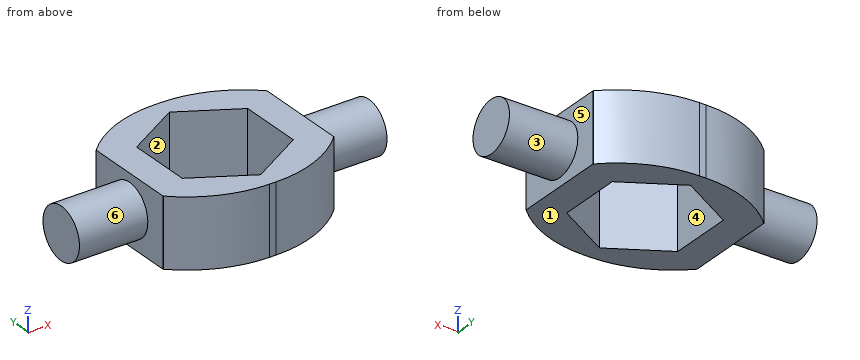
from build123d import *

# Parameters (mm, degrees)
SKETCH1_W           = 63.5
SKETCH1_H           = 60.360264722
BOSS_EXTRUDE1_DEPTH = 25.4
CHAMFER1_SIZE       = 12.7
SKETCH2_R           = 9.525
BOSS_EXTRUDE2_DEPTH = 25.4
FILLET1_R           = 43.18


with BuildPart() as part:
    # Sketch1 → Boss-Extrude1 (new body)
    with BuildSketch(Plane.XY):
        with Locations((31.75, 30.180132361)):
            Rectangle(SKETCH1_W, SKETCH1_H)
        Polygon((11.1125, 42.095198541), (11.1125, 18.26506618), (31.75, 6.35), (52.3875, 18.26506618), (52.3875, 42.095198541), (31.75, 54.010264722), align=None, mode=Mode.SUBTRACT)
    extrude(amount=BOSS_EXTRUDE1_DEPTH)

    # Chamfer1
    chamfer1_edges = [part.edges().sort_by_distance(p)[0] for p in [
        (0, 60.360264722, 12.7),
        (63.5, 60.360264722, 12.7),
        (63.5, 0, 12.7),
        (0, 0, 12.7),
    ]]
    chamfer(chamfer1_edges, length=CHAMFER1_SIZE)

    # Sketch2 → Boss-Extrude2 (add)
    with BuildSketch(Plane.ZY):
        with Locations((12.7, 30.180132361)):
            Circle(SKETCH2_R)
    boss_extrude2 = extrude(amount=BOSS_EXTRUDE2_DEPTH)

    # Mirror1: Boss-Extrude2 across plane
    add(boss_extrude2.mirror(Plane(origin=(31.75, 0, 0), x_dir=(0, 0, 1), z_dir=(1, 0, 0))))

    # Fillet1
    fillet1_edges = [part.edges().sort_by_distance(p)[0] for p in [
        (12.7, 60.360264722, 12.7),
        (50.8, 60.360264722, 12.7),
        (12.7, 0, 12.7),
        (50.8, 0, 12.7),
    ]]
    fillet(fillet1_edges, radius=FILLET1_R)


solid = part.part
Can you work these out from the model? Positions are in its coordinate system, mm. Face numbers are marked on the shaded views. A direction names the side the tool comes from. Give positions to 0.01 mm unless a question says otherwise; leave off trailing zeros. Loops run counter-clockwise (first coordinate to the right, second up) from the corner with the lowest first, then second, coordinate; pieces in that order, holes last. Notation, with made-up numbers: (37, -38) - (96, -38) arc R32 cw to (96, -8) - close; hole circle Ø11 at (-11.5, 52). An arc over 180 degrees is marked (long way). Return JSON: item names as keys, results as strings.
1. I want a section at B-B on x = 37. Please give me the cut outline in (y, z).
Output values:
{"outline": "(0.19, 0) - (9.38, 0) - (9.38, 25.4) - (0.19, 25.4) - close; (50.98, 0) - (60.17, 0) - (60.17, 25.4) - (50.98, 25.4) - close"}
2. I want a section at C-C on y = 25. Please give me the cut outline in (x, z), and give its area (3 significant figures).
Output values:
{"outline": "(-25.4, 4.71) - (0, 4.71) - (0, 0) - (11.11, 0) - (11.11, 25.4) - (0, 25.4) - (0, 20.69) - (-25.4, 20.69) - close; (52.39, 0) - (63.5, 0) - (63.5, 4.71) - (88.9, 4.71) - (88.9, 20.69) - (63.5, 20.69) - (63.5, 25.4) - (52.39, 25.4) - close", "area": "1,380 mm²"}
3. I want a section at D-D on z = 23.5. Please give me the cut outline in (x, y), and give its area (3 significant figures).
Output values:
{"outline": "(0, 12.7) - (0.05, 12.65) arc R43.18 ccw to (30.59, 0) - (32.91, 0) arc R43.18 ccw to (63.45, 12.65) - (63.5, 12.7) - (63.5, 47.66) - (63.45, 47.71) arc R43.18 ccw to (32.91, 60.36) - (30.59, 60.36) arc R43.18 ccw to (0.05, 47.71) - (0, 47.66) - close; hole (11.11, 18.27) - (31.75, 6.35) - (52.39, 18.27) - (52.39, 42.1) - (31.75, 54.01) - (11.11, 42.1) - close", "area": "1,870 mm²"}
4. I'm going to push flat-ended pins straight in: pin 1 Ø5 at (x, z) = (39, 14.5) entering from +Y; pin 2 Ø12 at (x, z) = (14.5, 4) entering from +Y; pin 3 Ø3 at (x, z) = (36, 15) entering from -Y; pin 4 Ø12 at (x, y) = (72, 13.5) entering from +Z. Where does each tip first touch, or does it pass through?
Output values:
{"pin 1": "stops at y = 60.21", "pin 2": "stops at y = 59.17", "pin 3": "stops at y = 0.03", "pin 4": "passes through"}
5. I want a section at A-A on z = 12.7. Please give me the cut outline in (x, y), and give its area (3 significant figures).
Output values:
{"outline": "(-25.4, 20.66) - (0, 20.66) - (0, 12.7) - (0.05, 12.65) arc R43.18 ccw to (30.59, 0) - (32.91, 0) arc R43.18 ccw to (63.45, 12.65) - (63.5, 12.7) - (63.5, 20.66) - (88.9, 20.66) - (88.9, 39.71) - (63.5, 39.71) - (63.5, 47.66) - (63.45, 47.71) arc R43.18 ccw to (32.91, 60.36) - (30.59, 60.36) arc R43.18 ccw to (0.05, 47.71) - (0, 47.66) - (0, 39.71) - (-25.4, 39.71) - close; hole (11.11, 18.27) - (31.75, 6.35) - (52.39, 18.27) - (52.39, 42.1) - (31.75, 54.01) - (11.11, 42.1) - close", "area": "2,840 mm²"}
6. For the marked faces 4, 5 and 6, which set-ups out of +Z, -Z, +X, -X, +Y, -Y let a thin tool reach every point of the face, with its end or its side?
Output values:
{"face 4": "+Z, -Z", "face 5": "+X", "face 6": "-X"}
7. We'd pull the mould along Y, two halves only. Please class the marked faces 1, 2 and 3: +Y half, -Y half, draft (parallel to the pull), parting line (faces both ways), or undercut.
Output values:
{"face 1": "draft", "face 2": "undercut", "face 3": "parting line"}
8. If I drill on line 1 (X direction, y = 18.5, z = 12.75); line 2 (X direction, y = 23.5, z = 9.25); line 3 (Y direction, x = 30, z = 14.25), over which ranges is the centre line in solid material (lowest first)?
Output values:
{"line 1": "x = 0 to 11.11, 52.39 to 63.5", "line 2": "x = -25.4 to 11.11, 52.39 to 88.9", "line 3": "y = 0 to 7.36, 53 to 60.36"}
